Check sheet for the drawn part. Datum: minimum x, y, z corner. Units: mm. A direction names the side the tool comes from. Round coordinates to 2 decimals unless told otherwise and drop trailing zeros. Write each loop counter-clockwise with the first axis right and the second up, starting at its lowest first coordinate (ties: lowest second). Pieces come first, ordered by that corner, then holes. Notation, with made-up numbers: M 27.5,66.25 L 85.5,66.25 A6 ccw 85.5,75.25 Z; hole C -33.75,14 d11. An arc over 180 degrees is marked long. Answer in a Markdown table with one row per item. Add a question column.
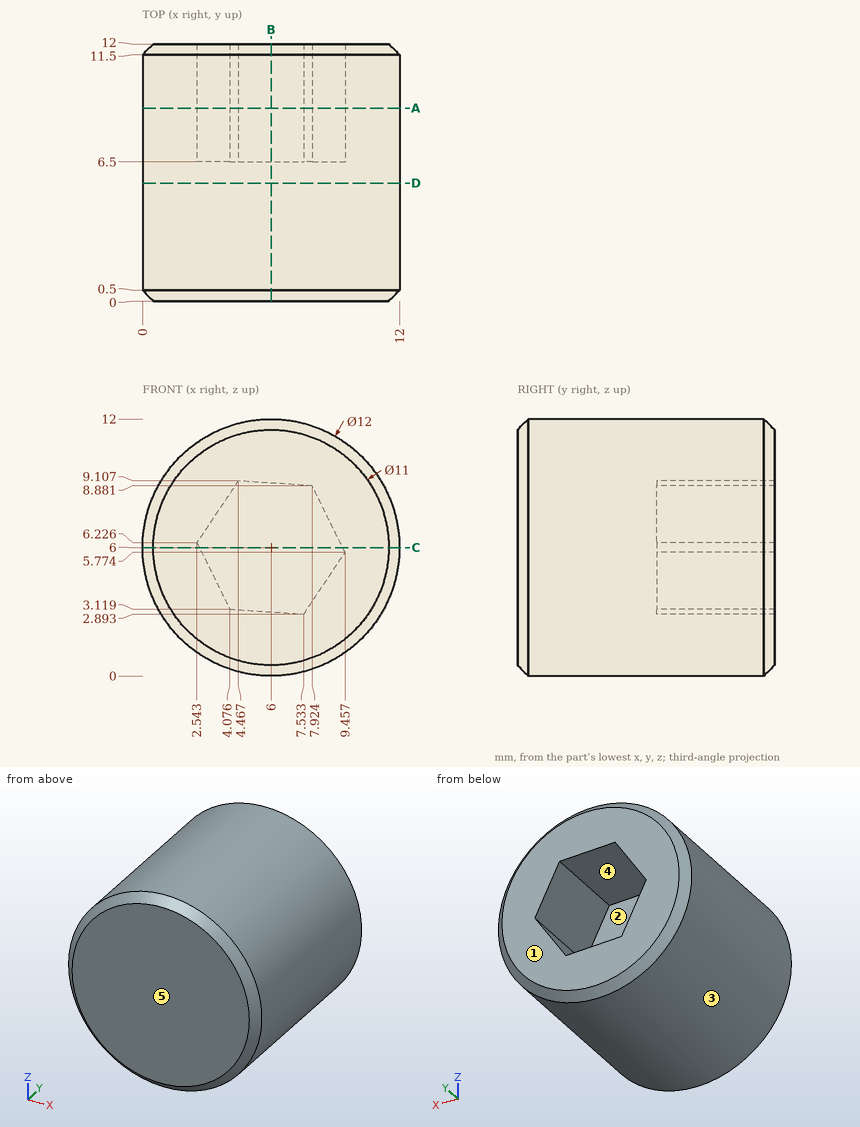
Item 1: Gauge pin test, flat ends, axial feed: pin 1 Ø1 at (y, z) = (6.5, 8) entering from -X; pin 2 Ø1.9 at (x, z) = (7, 6) entering from +Y. Record the tip position at first contact, or that the pin passes through.
Item 2: Mould release check, pull along Z, two halves, no side actions. Record for the marked faces 1, 2 and 3: +Z half, -Z half, draft (parallel to the pull), parting line (faces both ways), or undercut.
Item 3: Scan lines: probe 1 along Y at (x, z) = (5.5, 5.75); probe 2 along Z at (x, y) = (4.5, 7.75) (1 decimal); probe 3 along Z at (x, y) = (4.25, 10.5) (1 decimal). Record each from-to range of solid material in increasing order. Write a range as from..to.
Item 4: Section check C-C, the plane z = 6. Record the boundary of the cut face in (x, y) (1 decimal), and give its area (3 significant figures).
Item 5: Section check D-D, the plane y = 5.5. Record the boundary of the cut face in (x, z).
Item 6: Section check B-B, the plane x = 6. Record the boundary of the cut face in (y, z).
Item 7: Section check A-A, the plane y = 9. Record the boundary of the cut face in (x, z).
Item 8: Access from +Z, -Z, +X, -X, +Y, -Y to the whole of each face (thin tool, end or side, straight path). Record for the marked faces 4 and 5.
Result sheet:
| question | item | result |
|---|---|---|
| 1 | pin 1 | stops at x = 0.19 |
| 1 | pin 2 | stops at y = 6.5 |
| 2 | face 1 | draft |
| 2 | face 2 | undercut |
| 2 | face 3 | parting line |
| 3 | probe 1 | y = 0..6.5 |
| 3 | probe 2 | z = 0.2..3.1, 9.1..11.8 |
| 3 | probe 3 | z = 0.3..3.1, 8.8..11.7 |
| 4 | outline | M 0,0.5 L 0.5,0 L 11.5,0 L 12,0.5 L 12,11.5 L 11.5,12 L 9.3,12 L 9.3,6.5 L 2.7,6.5 L 2.7,12 L 0.5,12 L 0,11.5 Z |
| 4 | area | 107 mm^2 |
| 5 | outline | C 6,6 d12 |
| 6 | outline | M 0,0.5 L 0.5,0 L 11.5,0 L 12,0.5 L 12,2.99 L 6.5,2.99 L 6.5,9.01 L 12,9.01 L 12,11.5 L 11.5,12 L 0.5,12 L 0,11.5 Z |
| 7 | outline | C 6,6 d12; hole M 2.54,6.23 L 4.08,3.12 L 7.53,2.89 L 9.46,5.77 L 7.92,8.88 L 4.47,9.11 Z |
| 8 | face 4 | +Y |
| 8 | face 5 | +Z, -Z, +X, -X, -Y |
